```python
from build123d import *

# Parameters (mm, degrees)
FILLET1_R   = 0.1
HEX_2_DEPTH = 1.3


with BuildPart() as part:
    # BodySke → Base-Revolve (revolve)
    with BuildSketch(Plane.XY):
        Polygon((0, 0), (0, 2.45), (0.3, 2.75), (3, 2.75), (3, 1.5), (9.7195, 1.5), (10, 1.2195), (10, 0), align=None)
    revolve(axis=Axis((-31.75, 0, 0), (1, 0, 0)))

    # Fillet1
    fillet1_edges = [part.edges().sort_by_distance(p)[0] for p in [
        (3, -1.5, 0),
    ]]
    fillet(fillet1_edges, radius=FILLET1_R)

    # Sketch2 → Hex-PreBroach (revolve, cut)
    with BuildSketch(Plane.XY):
        Polygon((0, 1.28), (1.3, 1.28), (2.039008345, 0), (0, 0), align=None)
    revolve(axis=Axis((0, 0, 0), (1, 0, 0)), mode=Mode.SUBTRACT)

    # Sketch3 → Hex 2 (cut)
    with BuildSketch(Plane(origin=(0, 0, 0), x_dir=(0, 0.5, 0.866025404), z_dir=(-1, 0, 0))):
        Polygon((0.739008345, 1.28), (-0.739008345, 1.28), (-1.478016689, 0), (-0.739008345, -1.28), (0.739008345, -1.28), (1.478016689, 0), align=None)
    extrude(amount=-HEX_2_DEPTH, mode=Mode.SUBTRACT)


solid = part.part
```
The listing builds one solid part. Answer for the finished solid, in the listing's coordinates (mm). A direction names the side the tool comes from. Give positions to 0.01 mm unless a question says otherwise; leave off trailing zeros. Order: outer loops, then holes, each group sorted by start corner. A loop starts at its lowest first (then second) coordinate and runs counter-clockwise, first axis right, second up. Notation, with made-up numbers: (81, 73) - (88, 73) arc R20 ccw to (88, 96) - close; hole circle Ø5 at (47.5, 71.25). An arc over 180 degrees is marked (long way). Answer in a Markdown table with one row per item. Add a question column.
Q1. The part is cut by section A-A (x = 7.5). Determine the outline of the cut face in (y, z), then the cut area to 3 significant figures.
Q2. Given P1, Ø0.5, axis at y = 0.5, z = 1, coming from the -X side, flat-ended and moving along its own axis, determine where the tip first touches the part or whether it passes through.
Q3. For a pull along Y with two mould halves and no side action, classify faces 4 (the flat face through (0.641, 1.114, -0.631)), 5 (the flat face through (1, 0, -1.28)), 6 (the flat face through (10, 0, 0)), 7 (the cylindrical face through (1.669, -0.596, -2.685)) as released by +Y, released by -Y, zero draft, split by the parting line, or undercut.
Q4. Find the intervals of material crossed by line 1 along Y through (x, z) = (4.75, 0.25); line 2 along Z through (x, y) = (7, 0.1); line 3 along X through (y, z) = (1.3, -1.25), in increasing order. Write a range as [from, to].
Q5. Which of the six approach directions +Z, -Z, +X, -X, +Y, -Y give full straight-line access (tool end or side, diameter ignored) to faces 1 (the cylindrical face through (6.46, -1.5, 0.07)), 2 (the flat face through (0.641, -1.114, 0.631)), 3 (the flat face through (0, -1.1, -1.1))?
Determined:
| question | item | result |
|---|---|---|
| 1 | outline | circle Ø3 at (0, 0) |
| 1 | area | 7.07 mm² |
| 2 | P1 | stops at x = 1.3 |
| 3 | face 4 | undercut |
| 3 | face 5 | undercut |
| 3 | face 6 | zero draft |
| 3 | face 7 | split by the parting line |
| 4 | line 1 | y = [-1.48, 1.48] |
| 4 | line 2 | z = [-1.5, 1.5] |
| 4 | line 3 | x = [0, 3] |
| 5 | face 1 | +X |
| 5 | face 2 | -X |
| 5 | face 3 | +Z, -Z, -X, +Y, -Y |
